Autodesk Inventor part; units mm, degrees
ref_plane "YZ Plane" through (0, 0, 0) normal (1, 0, 0) x (0, 1, 0)
ref_plane "XZ Plane" through (0, 0, 0) normal (0, 1, 0) x (-1, 0, 0)
ref_plane "XY Plane" through (0, 0, 0) normal (0, 0, 1) x (1, 0, 0)
sketch "Sketch1" plane through (0, 0, 0) normal (0, 1, 0) x (-1, 0, 0)
  line L0 (0, 0) -> (-20.3, 0)
  line L1 (-20.3, 0) -> (-20.3, 10.3)
  line L2 (-20.3, 10.3) -> (0, 10.3)
  line L3 (0, 10.3) -> (0, 0)
  line L4 (-2.2, 2.2) -> (-18.1, 2.2)
  line L5 (-18.1, 2.2) -> (-18.1, 8.1)
  line L6 (-18.1, 8.1) -> (-2.2, 8.1)
  line L7 (-2.2, 8.1) -> (-2.2, 2.2)
  dimension "d0" = 20.3
  dimension "d1" = 10.3
  dimension "d2" = 2.2
extrude "Extrusion1" add sketch "Sketch1" along normal blind 150
extrude "Extrusion2" add sketch "Sketch1" against normal blind 25
properties part number "Beam" material "Aluminum 3004-O"
Geometry check sheet. Reference: the model listing, model coordinates, mm. A direction names the side the tool comes from. Give positions to 0.01 mm unless a question says otherwise; leave off trailing zeros. Order: outer loops, then holes, each group sorted by start corner. A loop starts at its lowest first (then second) coordinate and runs counter-clockwise, first axis right, second up.
1. Release check for a two-part mould opening along Z. For faces 3 (the face through (18.1, 61, 5)), 4 (the face through (20.3, 61, 5)), 5 (the face through (10, 61, 0)) record: pulls with the +Z half, pulls with the -Z half, needs draft (parallel to the pull), parting line crosses it, or undercut.
2. Access from +Z, -Z, +X, -X, +Y, -Y to the whole of each face (thin tool, end or side, straight path). Record for faces 1 (the face through (10, 61, 10.3)), 2 (the face through (10, 61, 2.2)).
3. Section check A-A, the plane z = 6. Enter the section's corners in (x, y).
4. Section check C-C, the plane y = 100.5. Enter the section's corners in (x, z), and give its area (3 significant figures).
5. Gauge pin test, flat end, axial feed: pin 1 Ø4 at (x, z) = (6, 4.5) entering from -Y. Record the tip position at first contact, or that the pin passes through.
6. Thickness scan on L1, parallel to X at y = 126, z = 3.5; L2, parallel to Z at x = 8.75, y = 1.5. Record the ranges inside material, lowest first.
7. Section check B-B, the plane x = 8.25. Enter the section's corners in (y, z), and give its area (3 significant figures).
Values follow:
1. face 3: undercut
1. face 4: needs draft
1. face 5: pulls with the -Z half
2. face 1: +Z, +X, -X, +Y, -Y
2. face 2: +Y, -Y
3. outline: (0, -25) - (2.2, -25) - (2.2, 150) - (0, 150) - close; (18.1, -25) - (20.3, -25) - (20.3, 150) - (18.1, 150) - close
4. outline: (0, 0) - (20.3, 0) - (20.3, 10.3) - (0, 10.3) - close; hole (2.2, 2.2) - (18.1, 2.2) - (18.1, 8.1) - (2.2, 8.1) - close
4. area: 115 mm2
5. pin 1: passes through
6. L1: x = 0 to 2.2, 18.1 to 20.3
6. L2: z = 0 to 2.2, 8.1 to 10.3
7. outline: (-25, 0) - (150, 0) - (150, 2.2) - (-25, 2.2) - close; (-25, 8.1) - (150, 8.1) - (150, 10.3) - (-25, 10.3) - close
7. area: 770 mm2
